from build123d import *

# Parameters (mm, degrees)
SKETCH1_W           = 44.1
SKETCH1_H           = 8
BOSS_EXTRUDE1_DEPTH = 2
SKETCH2_W           = 12
SKETCH2_H           = 2
BOSS_EXTRUDE2_DEPTH = 3
CUT_EXTRUDE1_DEPTH  = 46.097782651
SKETCH4_W           = 32.1
SKETCH4_H           = 2
BOSS_EXTRUDE3_DEPTH = 1
SKETCH7_R           = 2.794
CUT_EXTRUDE3_DEPTH  = 45.382541613
SKETCH8_R           = 1.5875
CUT_EXTRUDE4_DEPTH  = 45.382541613
BOSS_EXTRUDE4_DEPTH = 3


with BuildPart() as part:
    # Sketch1 → Boss-Extrude1 (new body)
    with BuildSketch(Plane(origin=(0, 0, 0), x_dir=(1, 0, 0), z_dir=(0, 1, 0))):
        with Locations((22.05, 0)):
            Rectangle(SKETCH1_W, SKETCH1_H)
    boss_extrude1 = extrude(amount=BOSS_EXTRUDE1_DEPTH)

    # Sketch2 → Boss-Extrude2 (add)
    with BuildSketch(Plane(origin=(0, 2, 0), x_dir=(1, 0, 0), z_dir=(0, 1, 0))):
        with Locations((38.1, 3)):
            Rectangle(SKETCH2_W, SKETCH2_H)
        with Locations((38.1, -3)):
            Rectangle(SKETCH2_W, SKETCH2_H)
    boss_extrude2 = extrude(amount=BOSS_EXTRUDE2_DEPTH)

    # Sketch3 → Cut-Extrude1 (cut, through all)
    with BuildSketch(Plane.XY.offset(4)):
        with BuildLine():
            Line((36.6, 3.5), (36.6, 5))
            Line((36.6, 5), (39.6, 5))
            Line((39.6, 5), (39.6, 3.5))
            ThreePointArc((39.6, 3.5), (38.1, 2), (36.6, 3.5))
        make_face()
    cut_extrude1 = extrude(amount=-CUT_EXTRUDE1_DEPTH, mode=Mode.SUBTRACT)

    # Sketch4 → Boss-Extrude3 (add)
    with BuildSketch(Plane(origin=(0, 2, 0), x_dir=(1, 0, 0), z_dir=(0, 1, 0))):
        with Locations((16.05, -3)):
            Rectangle(SKETCH4_W, SKETCH4_H)
        with Locations((16.05, 3)):
            Rectangle(SKETCH4_W, SKETCH4_H)
    boss_extrude3 = extrude(amount=BOSS_EXTRUDE3_DEPTH)

    # Mirror1: Boss-Extrude1, Boss-Extrude2, Cut-Extrude1, Boss-Extrude3 across plane
    add(boss_extrude1.mirror(Plane(origin=(0, 0, 0), x_dir=(0, 0, 1), z_dir=(1, 0, 0))))
    add(boss_extrude2.mirror(Plane(origin=(0, 0, 0), x_dir=(0, 0, 1), z_dir=(1, 0, 0))))
    add(cut_extrude1.mirror(Plane(origin=(0, 0, 0), x_dir=(0, 0, 1), z_dir=(1, 0, 0))), mode=Mode.SUBTRACT)
    add(boss_extrude3.mirror(Plane(origin=(0, 0, 0), x_dir=(0, 0, 1), z_dir=(1, 0, 0))))

    # Sketch7 → Cut-Extrude3 (cut, through all)
    with BuildSketch(Plane(origin=(0, 2, 0), x_dir=(1, 0, 0), z_dir=(0, 1, 0))):
        with Locations((10, 0)):
            Circle(SKETCH7_R)
    cut_extrude3 = extrude(amount=CUT_EXTRUDE3_DEPTH, mode=Mode.SUBTRACT)

    # Sketch8 → Cut-Extrude4 (cut, through all)
    with BuildSketch(Plane(origin=(0, 2, 0), x_dir=(1, 0, 0), z_dir=(0, 1, 0))):
        with Locations(Location((10, 0, 0), (0, 0, 270))):
            Circle(SKETCH8_R)
    cut_extrude4 = extrude(amount=-CUT_EXTRUDE4_DEPTH, mode=Mode.SUBTRACT)

    # Sketch9 → Boss-Extrude4 (add)
    with BuildSketch(Plane(origin=(0, 3, 0), x_dir=(1, 0, 0), z_dir=(0, 1, 0))):
        with BuildLine():
            Line((12.642429942, 4), (7.357570058, 4))
            ThreePointArc((7.357570058, 4), (10, 4.794), (12.642429942, 4))
        make_face()
        with BuildLine():
            Line((7.357570058, -4), (12.642429942, -4))
            ThreePointArc((12.642429942, -4), (10, -4.794), (7.357570058, -4))
        make_face()
    boss_extrude4 = extrude(amount=-BOSS_EXTRUDE4_DEPTH)

    # Mirror2: Cut-Extrude3, Cut-Extrude4, Boss-Extrude4 across plane
    add(cut_extrude3.mirror(Plane(origin=(0, 0, 0), x_dir=(0, 0, 1), z_dir=(1, 0, 0))), mode=Mode.SUBTRACT)
    add(cut_extrude4.mirror(Plane(origin=(0, 0, 0), x_dir=(0, 0, 1), z_dir=(1, 0, 0))), mode=Mode.SUBTRACT)
    add(boss_extrude4.mirror(Plane(origin=(0, 0, 0), x_dir=(0, 0, 1), z_dir=(1, 0, 0))))


solid = part.part
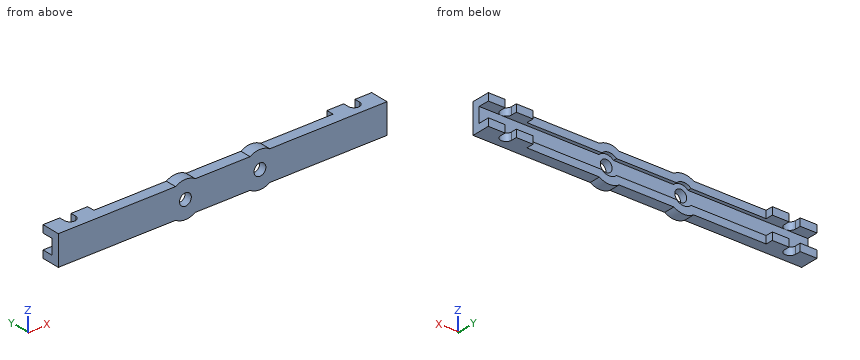
Could you check a few things on this model? Use its own coordinates, in mm. Coordinates: 2 decimals unless noted, no trailing zeros. Order: outer loops, then holes, each group sorted by start corner. A loop starts at its lowest first (then second) coordinate and runs counter-clockwise, first axis right, second up. Notation, with made-up numbers: (57.25, -14.5) - (110.25, -14.5) arc R22 cw to (110.25, -2.5) - close; hole circle Ø7 at (86.5, -11). An arc over 180 degrees is marked (long way). Answer in a Markdown table with one row per item. Add a question column.
(1) If we section it at D-D, the plane x = -26: Please give me the cut outline in (y, z).
(2) I need wall thicknesses on L1, parallel to X at y = 4.3, z = 2.75; L2, parallel to X at y = 0.8, z = 0; L3, parallel to Z at x = -10, y = 1.2. Which ranges of each line are inside material? Lowest first, please.
(3) If we section it at A-A, the plane x = -10: Please give me the cut outline in (y, z).
(4) If we section it at C-C, the plane y = 1.1: Please give me the cut outline in (x, z) (1 decimal).
(5) If we section it at B-B, the plane z = 0: Please give me the cut outline in (x, y).
(6) Will these pins go through, and if not, where does the flat tip stop? pin 1 (1.5 mm diameter, centred on x = -3, z = 2, fed in from +Y); pin 2 (2.5 mm diameter, centred on x = 27.5, y = 1.5, fed in from -Z); pin 3 (1.5 mm diameter, centred on x = 27.5, y = 2, fed in from +Z).
Results are:
| question | item | result |
|---|---|---|
| 1 | outline | (0, -4) - (3, -4) - (3, -2) - (2, -2) - (2, 2) - (3, 2) - (3, 4) - (0, 4) - close |
| 2 | L1 | x = -44.1 to -39.6, -36.6 to -32.1, 32.1 to 36.6, 39.6 to 44.1 |
| 2 | L2 | x = -44.1 to -11.59, -8.41 to 8.41, 11.59 to 44.1 |
| 2 | L3 | z = -4.79 to -1.59, 1.59 to 4.79 |
| 3 | outline | (0, -4.79) - (3, -4.79) - (3, -2.79) - (2, -2.79) - (2, -1.59) - (0, -1.59) - close; (0, 1.59) - (2, 1.59) - (2, 2.79) - (3, 2.79) - (3, 4.79) - (0, 4.79) - close |
| 4 | outline | (-44.1, -4) - (-12.6, -4) arc R4.8 ccw to (-7.4, -4) - (7.4, -4) arc R4.8 ccw to (12.6, -4) - (44.1, -4) - (44.1, 4) - (12.6, 4) arc R4.8 ccw to (7.4, 4) - (-7.4, 4) arc R4.8 ccw to (-12.6, 4) - (-44.1, 4) - close; hole circle Ø3.2 at (-10, 0); hole circle Ø3.2 at (10, 0) |
| 5 | outline | (-44.1, 0) - (-11.59, 0) - (-11.59, 2) - (-44.1, 2) - close; (-8.41, 0) - (8.41, 0) - (8.41, 2) - (-8.41, 2) - close; (11.59, 0) - (44.1, 0) - (44.1, 2) - (11.59, 2) - close |
| 6 | pin 1 | stops at y = 3 |
| 6 | pin 2 | stops at z = -4 |
| 6 | pin 3 | stops at z = 4 |
